Design review of the part shown in the three views and the two pictorial views. Dimensions are in mm from the part's minimum x, y and z. A direction names the side the tool comes from. Coordinates: 2 decimals unless noted, no trailing zeros. Write each loop counter-clockwise with the first axis right and the second up, starting at its lowest first coordinate (ties: lowest second). Pieces come first, ordered by that corner, then holes. Notation, with made-up numbers: M -23,-12.75 L -10,-12.75 A30 cw -10,17.25 Z; hole C -14.5,-20.5 d2. An arc over 180 degrees is marked long. One line per question, with ' | ' between items.
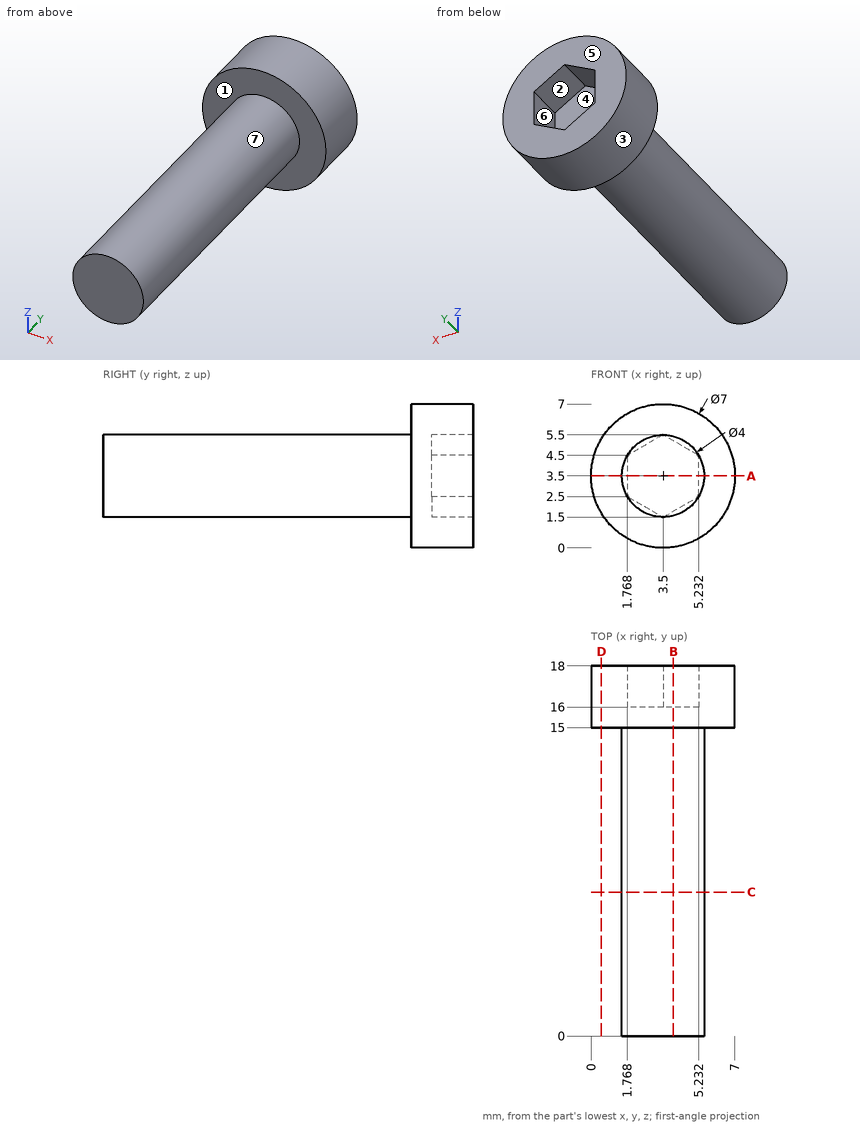
1. Take a section at B-B on x = 4. State the section outline as (y, z) points.
Computed values:
outline: M 0,1.56 L 15,1.56 L 15,0.04 L 18,0.04 L 18,1.79 L 16,1.79 L 16,5.21 L 18,5.21 L 18,6.96 L 15,6.96 L 15,5.44 L 0,5.44 Z
2. Draft analysis for pull direction X (two halves, no side actions). For the marked faces 1, 2, 3 and 4, state which applies: pulls with the +X half, pulls with the -X half, needs draft (parallel to the pull), parting line crosses it, or undercut.
Computed values:
face 1: needs draft | face 2: undercut | face 3: parting line crosses it | face 4: undercut
3. For line 1 along Y through (x, z) = (4.75, 1.5); line 2 along X through (y, z) = (12.5, 4.5); line 3 along Y through (x, z) = (3.5, 2), list the stretches that pass through material, from the lowest coordinate up.
Computed values:
line 1: y = 15 to 18 | line 2: x = 1.77 to 5.23 | line 3: y = 0 to 16
4. Take a section at C-C on y = 7. State the section outline as (x, z) points.
Computed values:
outline: C 3.5,3.5 d4
5. Take a section at D-D on x = 0.5. State the section outline as (y, z) points.
Computed values:
outline: M 15,1.7 L 18,1.7 L 18,5.3 L 15,5.3 Z
6. Take a section at A-A on z = 3.5. State the section outline as (x, y) points, plus the area to 3 significant figures.
Computed values:
outline: M 0,15 L 1.5,15 L 1.5,0 L 5.5,0 L 5.5,15 L 7,15 L 7,18 L 5.23,18 L 5.23,16 L 1.77,16 L 1.77,18 L 0,18 Z | area: 74.1 mm2
7. Clearance check with flat-ended pins moving along their axes: P1, Ø1.7, axis at x = 4, z = 4, coming from the +Y side; P2, Ø2, axis at y = 11, z = 2, coming from the +X side; P3, Ø2, axis at y = 10.5, z = 6, coming from the +X side. State where each tip first meets the part, or that it passes through.
Computed values:
P1: stops at y = 16 | P2: stops at x = 5.44 | P3: stops at x = 4.82
8. Machinability: for the marked faces 5, 6 and 7, which of the approach directions +Z, -Z, +X, -X, +Y, -Y give a long, thin tool a straight path to every point of the face, cutting with its end or side? Answer none if there is none.
Computed values:
face 5: +Z, -Z, +X, -X, +Y | face 6: +Y | face 7: -Y
